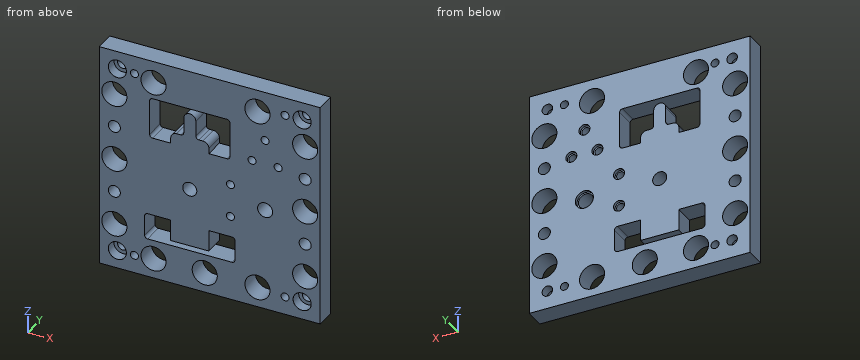
from build123d import *

# Parameters (mm, degrees)
SKETCH1_W                                    = 220
SKETCH1_H                                    = 225
BOSS_EXTRUDE1_DEPTH                          = 20
CUT_EXTRUDE3_REACH                           = 160.607
CUT_EXTRUDE4_REACH                           = 160.607
CUT_EXTRUDE5_REACH                           = 160.607
SKETCH7_R                                    = 4
CUT_EXTRUDE6_REACH                           = 160.607
SKETCH9_R                                    = 7.5
SKETCH10_R                                   = 5.5
CUT_EXTRUDE7_DEPTH                           = 3
SKETCH11_R                                   = 9
CUT_EXTRUDE8_DEPTH                           = 3
CBORE_FOR_M10_HEX_SOCKET_HEAD_CAP_SC_2_COUNT = 2
CBORE_FOR_M10_HEX_SOCKET_HEAD_CAP_SC_2_PITCH = 184
CBORE_FOR_M10_HEX_SOCKET_HEAD_CAP_SC_3_COUNT = 2
CBORE_FOR_M10_HEX_SOCKET_HEAD_CAP_SC_3_PITCH = 263.774524926
CBORE_FOR_M10_HEX_SOCKET_HEAD_CAP_SC_4_COUNT = 2
CBORE_FOR_M10_HEX_SOCKET_HEAD_CAP_SC_4_PITCH = 189
F_8_0MM_DOWEL_HOLE1_D                        = 8
F_25_0_25_DIAMETER_HOLE1_D                   = 25
CUT_EXTRUDE9_REACH                           = 160.607
SKETCH26_R                                   = 7
F_12_0_12_DIAMETER_HOLE1_D                   = 12


with BuildPart() as part:
    # Sketch1 → Boss-Extrude1 (new body)
    with BuildSketch(Plane(origin=(0, 0, 0), x_dir=(1, 0, 0), z_dir=(0, 1, 0))):
        Rectangle(SKETCH1_W, SKETCH1_H)
    extrude(amount=-BOSS_EXTRUDE1_DEPTH)

    # Sketch5 → Cut-Extrude3 (cut, up to next)
    with BuildSketch(Plane(origin=(0, 0, 0), x_dir=(1, 0, 0), z_dir=(0, 1, 0)), mode=Mode.PRIVATE) as cut_extrude3_sk1:
        with BuildLine():
            Line((-0.87, -38.14), (-0.87, -32.64))
            Line((-0.87, -32.64), (17.13, -32.64))
            ThreePointArc((17.13, -32.64), (19.251320344, -33.518679656), (20.13, -35.64))
            Line((20.13, -35.64), (20.13, -70.64))
            ThreePointArc((20.13, -70.64), (19.251320344, -72.761320344), (17.13, -73.64))
            Line((17.13, -73.64), (-56.87, -73.64))
            ThreePointArc((-56.87, -73.64), (-58.991320344, -72.761320344), (-59.87, -70.64))
            Line((-59.87, -70.64), (-59.87, -35.64))
            ThreePointArc((-59.87, -35.64), (-58.991320344, -33.518679656), (-56.87, -32.64))
            Line((-56.87, -32.64), (-38.87, -32.64))
            Line((-38.87, -32.64), (-38.87, -38.14))
            ThreePointArc((-38.87, -38.14), (-37.112640687, -42.382640687), (-32.87, -44.14))
            Line((-32.87, -44.14), (-28.87, -44.14))
            ThreePointArc((-28.87, -44.14), (-26.748679656, -45.018679656), (-25.87, -47.14))
            Line((-25.87, -47.14), (-25.87, -62.64))
            ThreePointArc((-25.87, -62.64), (-19.87, -68.64), (-13.87, -62.64))
            Line((-13.87, -62.64), (-13.87, -47.14))
            ThreePointArc((-13.87, -47.14), (-12.991320344, -45.018679656), (-10.87, -44.14))
            Line((-10.87, -44.14), (-6.87, -44.14))
            ThreePointArc((-6.87, -44.14), (-2.627359313, -42.382640687), (-0.87, -38.14))
        make_face()
    cut_extrude3_tool1 = extrude(cut_extrude3_sk1.sketch, amount=-CUT_EXTRUDE3_REACH, mode=Mode.PRIVATE) & part.part
    add(cut_extrude3_tool1.solids().sort_by_distance((-19.87, 0, 69.538944))[0], mode=Mode.SUBTRACT)

    # Sketch6 → Cut-Extrude4 (cut, up to next)
    with BuildSketch(Plane(origin=(0, 0, 0), x_dir=(1, 0, 0), z_dir=(0, 1, 0)), mode=Mode.PRIVATE) as cut_extrude4_sk1:
        with BuildLine():
            Line((-38.87, 47.36), (-61.87, 47.36))
            ThreePointArc((-61.87, 47.36), (-63.991320344, 48.238679656), (-64.87, 50.36))
            Line((-64.87, 50.36), (-64.87, 70.64))
            ThreePointArc((-64.87, 70.64), (-63.991320344, 72.761320344), (-61.87, 73.64))
            Line((-61.87, 73.64), (22.13, 73.64))
            ThreePointArc((22.13, 73.64), (24.251320344, 72.761320344), (25.13, 70.64))
            Line((25.13, 70.64), (25.13, 50.36))
            ThreePointArc((25.13, 50.36), (24.251320344, 48.238679656), (22.13, 47.36))
            Line((22.13, 47.36), (-0.87, 47.36))
            Line((-0.87, 47.36), (-0.87, 68.64))
            Line((-0.87, 68.64), (-38.87, 68.64))
            Line((-38.87, 68.64), (-38.87, 47.36))
        make_face()
    cut_extrude4_tool1 = extrude(cut_extrude4_sk1.sketch, amount=-CUT_EXTRUDE4_REACH, mode=Mode.PRIVATE) & part.part
    add(cut_extrude4_tool1.solids().sort_by_distance((-50.37, 0, -48.297584))[0], mode=Mode.SUBTRACT)

    # Sketch7 → Cut-Extrude5 (cut, up to next)
    with BuildSketch(Plane(origin=(0, 0, 0), x_dir=(1, 0, 0), z_dir=(0, 1, 0)), mode=Mode.PRIVATE) as cut_extrude5_sk1:
        with Locations(Location((55.13, -62.64, 0), (0, 0, 270))):
            Circle(SKETCH7_R)
    cut_extrude5_tool1 = extrude(cut_extrude5_sk1.sketch, amount=-CUT_EXTRUDE5_REACH, mode=Mode.PRIVATE) & part.part
    # Sketch7 → Cut-Extrude5 (cut, up to next)
    with BuildSketch(Plane(origin=(0, 0, 0), x_dir=(1, 0, 0), z_dir=(0, 1, 0)), mode=Mode.PRIVATE) as cut_extrude5_sk2:
        with Locations(Location((68.13, -38.14, 0), (0, 0, 270))):
            Circle(SKETCH7_R)
    cut_extrude5_tool2 = extrude(cut_extrude5_sk2.sketch, amount=-CUT_EXTRUDE5_REACH, mode=Mode.PRIVATE) & part.part
    # Sketch7 → Cut-Extrude5 (cut, up to next)
    with BuildSketch(Plane(origin=(0, 0, 0), x_dir=(1, 0, 0), z_dir=(0, 1, 0)), mode=Mode.PRIVATE) as cut_extrude5_sk3:
        with Locations(Location((42.13, -38.14, 0), (0, 0, 270))):
            Circle(SKETCH7_R)
    cut_extrude5_tool3 = extrude(cut_extrude5_sk3.sketch, amount=-CUT_EXTRUDE5_REACH, mode=Mode.PRIVATE) & part.part
    # Sketch7 → Cut-Extrude5 (cut, up to next)
    with BuildSketch(Plane(origin=(0, 0, 0), x_dir=(1, 0, 0), z_dir=(0, 1, 0)), mode=Mode.PRIVATE) as cut_extrude5_sk4:
        with Locations(Location((20.63, -6.64, 0), (0, 0, 270))):
            Circle(SKETCH7_R)
    cut_extrude5_tool4 = extrude(cut_extrude5_sk4.sketch, amount=-CUT_EXTRUDE5_REACH, mode=Mode.PRIVATE) & part.part
    # Sketch7 → Cut-Extrude5 (cut, up to next)
    with BuildSketch(Plane(origin=(0, 0, 0), x_dir=(1, 0, 0), z_dir=(0, 1, 0)), mode=Mode.PRIVATE) as cut_extrude5_sk5:
        with Locations(Location((20.63, 26.36, 0), (0, 0, 270))):
            Circle(SKETCH7_R)
    cut_extrude5_tool5 = extrude(cut_extrude5_sk5.sketch, amount=-CUT_EXTRUDE5_REACH, mode=Mode.PRIVATE) & part.part
    add(cut_extrude5_tool1.solids().sort_by_distance((55.13, 0, 62.64))[0], mode=Mode.SUBTRACT)
    add(cut_extrude5_tool2.solids().sort_by_distance((68.13, 0, 38.14))[0], mode=Mode.SUBTRACT)
    add(cut_extrude5_tool3.solids().sort_by_distance((42.13, 0, 38.14))[0], mode=Mode.SUBTRACT)
    add(cut_extrude5_tool4.solids().sort_by_distance((20.63, 0, 6.64))[0], mode=Mode.SUBTRACT)
    add(cut_extrude5_tool5.solids().sort_by_distance((20.63, 0, -26.36))[0], mode=Mode.SUBTRACT)

    # Sketch9 → Cut-Extrude6 (cut, up to next)
    with BuildSketch(Plane(origin=(0, 0, 0), x_dir=(1, 0, 0), z_dir=(0, 1, 0)), mode=Mode.PRIVATE) as cut_extrude6_sk1:
        with Locations(Location((55.13, 9.86, 0), (0, 0, 270))):
            Circle(SKETCH9_R)
    cut_extrude6_tool1 = extrude(cut_extrude6_sk1.sketch, amount=-CUT_EXTRUDE6_REACH, mode=Mode.PRIVATE) & part.part
    add(cut_extrude6_tool1.solids().sort_by_distance((55.13, 0, -9.86))[0], mode=Mode.SUBTRACT)

    # Sketch10 → Cut-Extrude7 (cut)
    with BuildSketch(Plane(origin=(0, 0, 0), x_dir=(1, 0, 0), z_dir=(0, 1, 0))):
        with Locations(Location((20.63, 26.36, 0), (0, 0, 270))):
            Circle(SKETCH10_R)
        with Locations(Location((20.63, -6.64, 0), (0, 0, 270))):
            Circle(SKETCH10_R)
        with Locations(Location((42.13, -38.14, 0), (0, 0, 270))):
            Circle(SKETCH10_R)
        with Locations(Location((68.13, -38.14, 0), (0, 0, 270))):
            Circle(SKETCH10_R)
        with Locations(Location((55.13, -62.64, 0), (0, 0, 270))):
            Circle(SKETCH10_R)
    extrude(amount=-CUT_EXTRUDE7_DEPTH, mode=Mode.SUBTRACT)

    # Sketch11 → Cut-Extrude8 (cut)
    with BuildSketch(Plane(origin=(0, 0, 0), x_dir=(1, 0, 0), z_dir=(0, 1, 0))):
        with Locations(Location((55.13, 9.86, 0), (0, 0, 270))):
            Circle(SKETCH11_R)
    extrude(amount=-CUT_EXTRUDE8_DEPTH, mode=Mode.SUBTRACT)

    # Sketch16 → CBORE for M10 Hex Socket Head Cap Screw1 (revolve, cut)
    with BuildSketch(Plane(origin=(92, -20, -94.5), x_dir=(0, 0, -1), z_dir=(1, 0, 0))):
        Polygon((0, 0), (0, 20), (5.25, 20), (5.25, 10.6), (9, 10.6), (9, 0.025), (9.025, 0), align=None)
    cbore_for_m10_hex_socket_head_cap_screw1 = revolve(axis=Axis((92, -26.35, -94.5), (0, 1, 0)), mode=Mode.SUBTRACT)

    # CBORE for M10 Hex Socket Head Cap Sc 2: CBORE for M10 Hex Socket Head Cap Screw1 ×2
    with Locations(*[(-i * CBORE_FOR_M10_HEX_SOCKET_HEAD_CAP_SC_2_PITCH, 0, 0) for i in range(1, CBORE_FOR_M10_HEX_SOCKET_HEAD_CAP_SC_2_COUNT)]):
        add(cbore_for_m10_hex_socket_head_cap_screw1, mode=Mode.SUBTRACT)

    # CBORE for M10 Hex Socket Head Cap Sc 3: CBORE for M10 Hex Socket Head Cap Screw1 ×2
    with Locations(*[Vector(-0.6975654682783963, 0, 0.7165210516555266) * (i * CBORE_FOR_M10_HEX_SOCKET_HEAD_CAP_SC_3_PITCH) for i in range(1, CBORE_FOR_M10_HEX_SOCKET_HEAD_CAP_SC_3_COUNT)]):
        add(cbore_for_m10_hex_socket_head_cap_screw1, mode=Mode.SUBTRACT)

    # CBORE for M10 Hex Socket Head Cap Sc 4: CBORE for M10 Hex Socket Head Cap Screw1 ×2
    with Locations(*[(0, 0, i * CBORE_FOR_M10_HEX_SOCKET_HEAD_CAP_SC_4_PITCH) for i in range(1, CBORE_FOR_M10_HEX_SOCKET_HEAD_CAP_SC_4_COUNT)]):
        add(cbore_for_m10_hex_socket_head_cap_screw1, mode=Mode.SUBTRACT)

    # 8.0mm Dowel Hole1 (through all)
    with Locations(Plane(origin=(0, -20, 0), x_dir=(-1, 0, 0), z_dir=(0, -1, 0))):
        with Locations((-75, 94.5), (75, 94.5), (75, -94.5), (-75, -94.5)):
            Hole(F_8_0MM_DOWEL_HOLE1_D / 2)

    # 25.0 _25_ Diameter Hole1 (through all)
    with Locations(Plane(origin=(0, 0, 0), x_dir=(1, 0, 0), z_dir=(0, 1, 0))):
        with Locations((-56, 92.5), (-5, 92.5), (47.5, 92.5), (95, 67.5), (95, 0), (95, -67.5), (47.5, -90.5), (-56, -90.5), (-95, -67.5), (-95, 0), (-95, 67.5)):
            Hole(F_25_0_25_DIAMETER_HOLE1_D / 2)

    # Sketch26 → Cut-Extrude9 (cut, up to next)
    with BuildSketch(Plane(origin=(0, 0, 0), x_dir=(1, 0, 0), z_dir=(0, 1, 0)), mode=Mode.PRIVATE) as cut_extrude9_sk1:
        with Locations(Location((-19.87, 9.86, 0), (0, 0, 270))):
            Circle(SKETCH26_R)
    cut_extrude9_tool1 = extrude(cut_extrude9_sk1.sketch, amount=-CUT_EXTRUDE9_REACH, mode=Mode.PRIVATE) & part.part
    add(cut_extrude9_tool1.solids().sort_by_distance((-19.87, 0, -9.86))[0], mode=Mode.SUBTRACT)

    # 12.0 _12_ Diameter Hole1 (through all)
    with Locations(Plane(origin=(0, 0, 0), x_dir=(1, 0, 0), z_dir=(0, 1, 0))):
        with Locations((95, 33.75), (-95, 33.75), (-95, -33.75), (95, -33.75)):
            Hole(F_12_0_12_DIAMETER_HOLE1_D / 2)


solid = part.part
Can you work these out from the model? Positions are in its coordinate system, mm. Give positions to 0.01 mm unless a question says otherwise; leave off trailing zeros. Order: outer loops, then holes, each group sorted by start corner. A loop starts at its lowest first (then second) coordinate and runs counter-clockwise, first axis right, second up. Notation, with made-up numbers: M 51,-9.5 L 79,-9.5 A21 ccw 79,16.5 Z; hole C 37,30.5 d10. An arc over 180 degrees is marked long. One line per question, with ' | ' between items.
Item 1: Suppose I cut it at A-A, the plane z = -63. Write out the boundary of the cut face in (x, y), then the cut area to 3 significant figures.
Answer block:
outline: M -110,-20 L -106.66,-20 L -106.66,0 L -110,0 Z; M -83.34,-20 L -64.87,-20 L -64.87,0 L -83.34,0 Z; M -38.87,-20 L -0.87,-20 L -0.87,0 L -38.87,0 Z; M 25.13,-20 L 83.34,-20 L 83.34,0 L 25.13,0 Z; M 106.66,-20 L 110,-20 L 110,0 L 106.66,0 Z | area: 2,430 mm2
Item 2: Please list where these lines run through material, in increasing order: L1, parallel to Z at x = 75, y = -8.5; L2, parallel to X at y = -15, z = -67.5; L3, parallel to Z at x = 8, y = -11.25.
Answer block:
L1: z = -112.5 to -98.5, -90.5 to 90.5, 98.5 to 112.5 | L2: x = -110 to -107.5, -82.5 to -64.87, -38.87 to -0.87, 25.13 to 82.5, 107.5 to 110 | L3: z = -112.5 to -73.64, -47.36 to 32.64, 73.64 to 112.5
Item 3: Suppose I cut it at B-B, the plane y = -13. Give the number of separate pieces and of enclosed holes in the cut face, then the cut area to 3 significant figures.
Answer block:
separate pieces: 1 | enclosed holes: 32 | area: 37,700 mm2
Item 4: I'm going to push a flat-ended pin straight in: pin 1 Ø14.5 at (x, z) = (92, 94.5) entering from -Y. Where does the tip first touch, or does it pass through?
Answer block:
pin 1: stops at y = -9.4
Item 5: Suppose I cut it at D-D, the plane z = -9.86. Write out the boundary of the cut face in (x, y).
Answer block:
outline: M -110,-20 L -102.68,-20 L -102.68,0 L -110,0 Z; M -87.32,-20 L -26.87,-20 L -26.87,0 L -87.32,0 Z; M -12.87,-20 L 47.63,-20 L 47.63,-3 L 46.13,-3 L 46.13,0 L -12.87,0 Z; M 62.63,-20 L 87.32,-20 L 87.32,0 L 64.13,0 L 64.13,-3 L 62.63,-3 Z; M 102.68,-20 L 110,-20 L 110,0 L 102.68,0 Z
